from build123d import *

# Parameters (mm, degrees)
F0_W     = 100.076
F0_H     = 2.54
F1_DEPTH = 11.938
F0_H_2   = 69.85
F2_DEPTH = 2.54
F4_DEPTH = 14.478
F5_W     = 13.97
F5_H     = 2.54
F6_DEPTH = 19.05
F7_R     = 2.5399
F3_R     = 1.524
F8_DEPTH = 76.2


# Not quite as in the source:
# - a fillet or chamfer is up to 0.001 mm smaller than in the source, because OpenCascade refuses the exact size


with BuildPart() as f1:
    # F0 (on Top) → F1 (new body)
    with BuildSketch(Plane.XY):
        with Locations((50.038, 71.12)):
            Rectangle(F0_W, F0_H)
    extrude(amount=F1_DEPTH)



with BuildPart() as f1b:
    # F0 (on Top) → F1, piece 2 (new body)
    with BuildSketch(Plane.XY):
        with Locations((50.038, -1.27)):
            Rectangle(F0_W, F0_H)
    extrude(amount=F1_DEPTH)


with BuildPart() as f1_1:
    add(f1.part)

    add(f1b.part)  # F2 merges F1b
    # F0 (on Top) → F2 (join)
    with BuildSketch(Plane.XY):
        with Locations((50.038, 34.925)):
            Rectangle(F0_W, F0_H_2)
    extrude(amount=F2_DEPTH)

    # F0 (on Top) → F4 (join)
    with BuildSketch(Plane.XY):
        Polygon((0, -2.54), (0, 0), (0, 69.85), (0, 72.39), (-2.54, 72.39), (-2.54, -2.54), align=None)
    extrude(amount=F4_DEPTH)

    # F5 (on face) → F6 (join)
    with BuildSketch(Plane(origin=(-2.54, 0, 0), x_dir=(0, -1, 0), z_dir=(-1, 0, 0))):
        with Locations((-34.925, 13.208)):
            Rectangle(F5_W, F5_H)
    extrude(amount=F6_DEPTH)

    # F7 (radius 2.54 in the source; OpenCascade refuses exactly that, so slightly less here)
    f7_edges = [f1_1.edges().sort_by_distance(p)[0] for p in [
        (-21.59, 27.94, 13.208),
        (-21.59, 41.91, 13.208),
        (-2.54, 41.91, 13.208),
        (-2.54, 27.94, 13.208),
        (-2.54, -2.54, 7.239),
        (100.076, -2.54, 5.969),
        (100.076, 72.39, 5.969),
        (-2.54, 72.39, 7.239),
        (0, 71.12, 11.938),
        (0, -1.27, 11.938),
        (-2.54, 34.925, 11.938),
    ]]
    fillet(f7_edges, radius=F7_R)

    # F3 (on face) → F8 (cut)
    with BuildSketch(Plane.XZ.offset(2.54)):
        with Locations((86.106, 6.604)):
            Circle(F3_R)
        with Locations((11.938, 6.604)):
            Circle(F3_R)
    extrude(amount=-F8_DEPTH, mode=Mode.SUBTRACT)


solid = f1_1.part
The listing builds one solid part. Answer for the finished solid, in the listing's coordinates (mm). A direction names the side the tool comes from. Coordinates: 2 decimals unless noted, no trailing zeros. Loops run counter-clockwise (first coordinate to the right, second up) from the corner with the lowest first, then second, coordinate; pieces in that order, holes last. Notation, with made-up numbers: (31, 56.25) -> (82, 56.25) arc R10 cw to (82, 65.25) -> close; hole circle Ø8 at (49.5, 46.25). An arc over 180 degrees is marked (long way). Write item = value, one per line. Start each with the question number.
1) The mould has two halves that part along Y. Classify faces 4 (the face through (-12, 27.94, 13)), 5 (the face through (49, 0, 7)), 6 (the face through (-21.59, 35, 13)): released by +Y, released by -Y, zero draft, split by the parting line, or undercut.
2) A cutting plane is placed at B-B (x = 47). Give the vertices of the cut face in (y, z), then the cut area to 3 significant figures.
3) A cutting plane is placed at A-A (y = 15). Give the vertices of the cut face in (x, z).
4) A cutting plane is placed at C-C (x = -10). Give the vertices of the cut face in (y, z).
5) Straight lines are drawn through the part: line 1 (Y direction, x = 28.5, z = 2.75); line 2 (X direction, y = 55.5, z = 3.5). For each, find the intervals that lie inside material, in ascending order. Write a range as from..to.
6) Given pin 1 Ø21 at (x, y) = (34.5, 22) entering from +Z; pin 2 Ø1.3 at (x, z) = (-13.5, 13.5) entering from +Y; pin 3 Ø3 at (x, y) = (61.5, 70.5) entering from +Z, each flat-ended and moving along its own axis, determine where each tip first touches the part or whether it passes through.
7) A tool of negligible diameter and unlimited length cuts with its end or side. For faces 1 (the face through (0, 34, 8)), 2 (the face through (-2.54, 35, 7)), 3 (the face through (51, 71, 11.938)), from which of +Z, -Z, +X, -X, +Y, -Y can it reach the whole face along a straight path? Write none if from no direction.
Responses:
q1.face_4 = released by -Y
q1.face_5 = undercut
q1.face_6 = zero draft
q2.outline = (-2.54, 0) -> (72.39, 0) -> (72.39, 11.94) -> (69.85, 11.94) -> (69.85, 2.54) -> (0, 2.54) -> (0, 11.94) -> (-2.54, 11.94) -> close
q2.area = 238 mm²
q3.outline = (-2.54, 0) -> (100.08, 0) -> (100.08, 2.54) -> (0, 2.54) -> (0, 14.48) -> (-2.54, 14.48) -> close
q4.outline = (27.94, 11.94) -> (41.91, 11.94) -> (41.91, 14.48) -> (27.94, 14.48) -> close
q5.line_1 = -2.54..0, 69.85..72.39
q5.line_2 = -2.54..0
q6.pin_1 = 2.54
q6.pin_2 = 41.91
q6.pin_3 = 11.94
q7.face_1 = +Z, +X
q7.face_2 = -Z, -X
q7.face_3 = +Z, +X, +Y, -Y
